```python
from build123d import *

# Parameters (mm, degrees)
F1_DEPTH     = 22
F2_R         = 1
F3_T1_DEPTH  = 31.8493182741
F3_T3_DEPTH  = 27.4759989859
F3_T8_DEPTH  = 1
F3_T14_DEPTH = 1
F4_R         = 1
F6_W         = 20.563358571
F6_H         = 20
F7_DEPTH     = 25
F9_D         = 4


# Not quite as in the source:
# - a fillet or chamfer that OpenCascade refuses, or shapes differently, is made with other operations: its cross-section is extruded or revolved along the edge and cut away or added


with BuildPart() as f1:
    # F0 (on Top) → F1 (new body)
    with BuildSketch(Plane.XY):
        Polygon((-24.8821492983, 2.4245919862), (0, 0), (-24.8821492983, 27.4245919862), align=None)
    extrude(amount=F1_DEPTH)

    # F2
    f2_edges = [f1.edges().sort_by_distance(p)[0] for p in [
        (-24.882149, 14.924592, 22),
        (-12.441075, 1.212296, 22),
    ]]
    fillet(f2_edges, radius=F2_R)

    # F3: fillet of radius 1 on 1 edges, made by hand

    # F3_s2 → F3_t1 (cut)
    with BuildSketch(Plane(origin=(-1.7406023493, 1.9184560251, 0), x_dir=(0, 0, 1), z_dir=(-0.6719435693, 0.7406023493, 0))):
        with BuildLine():
            ThreePointArc((21, 0), (21.7071067812, -0.2928932188), (22, -1))
            Line((22, -1), (22, 0))
            Line((22, 0), (21, 0))
        make_face()
    extrude(amount=F3_T1_DEPTH, mode=Mode.SUBTRACT)

    # F3_s4 → F3_t3 (cut)
    with BuildSketch(Plane.XY.offset(-6.4759989859)):
        with BuildLine():
            ThreePointArc((-24.8821492983, 24.8341923918), (-24.2422865296, 25.7670917297), (-23.141546949, 25.5061359611))
            Line((-23.141546949, 25.5061359611), (-24.8821492983, 27.4245919862))
            Line((-24.8821492983, 27.4245919862), (-24.8821492983, 24.8341923918))
        make_face()
        with BuildLine():
            ThreePointArc((-1.7406023493, 1.9184560251), (-1.5876305081, 0.7975969112), (-2.578188378, 0.2512264839))
            Line((-2.578188378, 0.2512264839), (0, 0))
            Line((0, 0), (-1.7406023493, 1.9184560251))
        make_face()
    extrude(amount=F3_T3_DEPTH, mode=Mode.SUBTRACT)


with BuildPart() as f3_tool6:
    # F3_s7 → F3_t8 (new body)
    with BuildSketch(Plane.XY.offset(21)):
        Polygon((-2.4812046985, 1.2465124558), (-1.7406023493, 1.9184560251), (0, 0), (-2.578188378, 0.2512264839), align=None)
    extrude(amount=F3_T8_DEPTH)

    # F3_s9 → F3_t10 (revolve, cut)
    with BuildSketch(Plane(origin=(-2.4812046985, 1.2465124558, 21), x_dir=(-0.8935741904, 0.4489155446, 0), z_dir=(0.4489155446, 0.8935741904, 0))):
        with BuildLine():
            ThreePointArc((0, -1), (1, 0), (0, 1))
            Line((0, 1), (0, -1))
        make_face()
    revolve(axis=Axis((-2.4812046985, 1.2465124558, 21), (0, 0, 1)), mode=Mode.SUBTRACT)


with BuildPart() as f1_1:
    add(f1.part)

    # F3_t5: cut F3_tool6
    add(f3_tool6.part, mode=Mode.SUBTRACT)


with BuildPart() as f3_tool12:
    # F3_s13 → F3_t14 (new body)
    with BuildSketch(Plane.XY.offset(21)):
        Polygon((-23.8821492983, 24.8341923918), (-24.8821492983, 24.8341923918), (-24.8821492983, 27.4245919862), (-23.141546949, 25.5061359611), align=None)
    extrude(amount=F3_T14_DEPTH)

    # F3_s15 → F3_t16 (revolve, cut)
    with BuildSketch(Plane(origin=(-23.8821492983, 24.8341923918, 21), x_dir=(0.3601372313, -0.9328993379, 0), z_dir=(-0.9328993379, -0.3601372313, 0))):
        with BuildLine():
            ThreePointArc((0, -1), (1, 0), (0, 1))
            Line((0, 1), (0, -1))
        make_face()
    revolve(axis=Axis((-23.8821492983, 24.8341923918, 21), (0, 0, 1)), mode=Mode.SUBTRACT)


with BuildPart() as f1_2:
    add(f1_1.part)

    # F3_t11: cut F3_tool12
    add(f3_tool12.part, mode=Mode.SUBTRACT)

    # F4
    f4_edges = [f1_2.edges().sort_by_distance(p)[0] for p in [
        (-13.730169, 1.337909, 0),
    ]]
    fillet(f4_edges, radius=F4_R)

    # F6 (on offset) → F7 (cut)
    with BuildSketch(Plane.XZ.offset(-3)):
        with Locations((-12.8598676635, 11)):
            Rectangle(F6_W, F6_H)
    extrude(amount=-F7_DEPTH, mode=Mode.SUBTRACT)

    # F9 (through all)
    with Locations(Plane(origin=(0, 3, 0), x_dir=(-1, 0, 0), z_dir=(0, 1, 0))):
        with Locations((12.000261806, 11.7051936686)):
            Hole(F9_D / 2)


solid = f1_2.part
```
For this review, take the finished solid that the model builds, in its own axes (mm). A direction names the side the tool comes from. Coordinates: 2 decimals unless noted, no trailing zeros. Loops run counter-clockwise (first coordinate to the right, second up) from the corner with the lowest first, then second, coordinate; pieces in that order, holes last.
1. For line 1 (Z direction, x = -21.5, y = 11.5); line 2 (Y direction, x = -19.75, z = 16.75); line 3 (X direction, y = 8.5, z = 11.25), list the stretches that pass through material, from the lowest coordinate up.
2. Mouldability with a two-part tool opening along Z and no side actions: class faces 1 (the cylindrical face through (-10.093, 1.973, 12.306)), 2 (the cylindrical face through (-24.597, 13.473, 0.301)), 3 (the cylindrical face through (-13.5, 1.6, 21.7)) as +Z half, -Z half, draft (parallel to the pull), parting line (faces both ways), or undercut.
3. Add section A-A, the plane z = 11. Give the boundary of the cut face in (x, y), then the cut area to 3 significant figures.
4. For faces 4 (the cylindrical face through (-12.802, 13.686, 0.301)), 5 (the flat face through (-13, 3, 9)), list the 3-axis set-ups (+Z, -Z, +X, -X, +Y, -Y) from which the entire face can be reached by the end or side of a thin tool; tool diameter is ignored.
5. Insertion check: P1, Ø12, axis at x = -10.5, z = 8, coming from the +Y side; P2, Ø3, axis at x = -20, z = 17, coming from the -Y side; P3, Ø8, axis at x = -22, y = 3, coming from the +Z side. Each pin has a flat end and moves straight along its axis. Give the tip position at first contact, or say it passes through.
6. Add section B-B, the plane z = 7.75. Give the boundary of the cut face in (x, y).
Result:
1. line 1: z = 0 to 1, 21 to 22
1. line 2: y = 1.92 to 3
1. line 3: x = -24.88 to -23.14
2. face 1: undercut
2. face 2: -Z half
2. face 3: +Z half
3. outline: (-24.88, 2.42) - (-13.87, 1.35) - (-13.87, 3) - (-23.14, 3) - (-23.14, 25.51) arc R1 ccw to (-24.88, 24.83) - close; (-10.13, 0.99) - (-2.58, 0.25) arc R1 ccw to (-1.74, 1.92) - (-2.72, 3) - (-10.13, 3) - close
3. area: 71.6 mm2
4. face 4: -Z, +X, +Y
4. face 5: +X, +Y
5. P1: stops at y = 3
5. P2: stops at y = 1.8
5. P3: stops at z = 22
6. outline: (-24.88, 2.42) - (-2.58, 0.25) arc R1 ccw to (-1.74, 1.92) - (-2.72, 3) - (-23.14, 3) - (-23.14, 25.51) arc R1 ccw to (-24.88, 24.83) - close
